```python
from build123d import *

# Parameters (mm, degrees)
F0_W     = 76.2336051654
F0_H     = 12.8238399291
F1_DEPTH = 25.4


with BuildPart() as f1:
    # F0 (on Front) → F1 (new body)
    with BuildSketch(Plane.XZ):
        with BuildLine():
            Line((0, -39.2335951328), (0, -55.1777966321))
            ThreePointArc((0, -55.1777966321), (25.3947344291, -51.0934089949), (48.2183970243, -39.2335951328))
            Line((48.2183970243, -39.2335951328), (0, -39.2335951328))
        make_face()
        Polygon((-74.7671502275, -55.1777966321), (0, -55.1777966321), (0, -39.2335951328), (-76.2336051654, -39.2335951328), (-76.2336051654, -55.1777966321), align=None)
        with BuildLine():
            Line((0, -39.2335951328), (48.2183970243, -39.2335951328))
            ThreePointArc((48.2183970243, -39.2335951328), (55.4027211148, -33.2174165852), (61.8420272475, -26.4097552037))
            Line((61.8420272475, -26.4097552037), (0, -26.4097552037))
            Line((0, -26.4097552037), (0, -39.2335951328))
        make_face()
        with BuildLine():
            ThreePointArc((-76.2336051654, -39.2335951328), (-97.2315440125, -49.2044021928), (-74.7671502275, -55.1777966321))
            Line((-74.7671502275, -55.1777966321), (-76.2336051654, -55.1777966321))
            Line((-76.2336051654, -55.1777966321), (-76.2336051654, -39.2335951328))
        make_face()
        with Locations((-38.1168025827, -32.8216751683)):
            Rectangle(F0_W, F0_H)
        with BuildLine():
            Line((61.8420272475, -13.3770994993), (61.8420272475, -26.4097552037))
            ThreePointArc((61.8420272475, -26.4097552037), (70.4948614625, -13.9048920781), (76.6509249806, 0))
            Line((76.6509249806, 0), (61.8420272475, 0))
            Line((61.8420272475, 0), (61.8420272475, -13.3770994993))
        make_face()
        Polygon((0, -26.4097552037), (61.8420272475, -26.4097552037), (61.8420272475, -13.3770994993), (0.0163518326, -13.2999842622), align=None)
        Polygon((-76.2336051654, -26.4097552037), (0, -26.4097552037), (0.0163518326, -13.2999842622), (-76.2336051654, -13.2048776019), align=None)
        Polygon((0.0163518326, -13.2999842622), (61.8420272475, -13.3770994993), (61.8420272475, 0), (21.9261534512, 0), (0.0329409185, 0), align=None)
        with BuildLine():
            ThreePointArc((-98.4511649107, 0), (-90.3999949354, -15.7771328177), (-76.2336051654, -26.4097552037))
            Line((-76.2336051654, -26.4097552037), (-76.2336051654, -13.2048776019))
            Line((-76.2336051654, -13.2048776019), (-76.2336051654, 0))
            Line((-76.2336051654, 0), (-78.4630104899, 0))
            Line((-78.4630104899, 0), (-98.4511649107, 0))
        make_face()
        Polygon((-76.2336051654, -13.2048776019), (0.0163518326, -13.2999842622), (0.0329409185, 0), (0, 0), (-20.4764902592, 0), (-61.0670559108, 0), (-76.2336051654, 0), align=None)
        Polygon((0.0329409185, 25.6056360344), (0.0329409185, 0), (21.9261534512, 0), (21.9261534512, 60.3007838378), (0.0329409185, 60.3007838378), align=None)
        Polygon((0, 0), (0.0329409185, 0), (0.0329409185, 25.6056360344), (-20.4764902592, 25.6056360344), (-20.4764902592, 0), align=None)
        Polygon((-78.4630104899, 0), (-76.2336051654, 0), (-61.0670559108, 0), (-61.0670559108, 8.4261661395), (-78.4630104899, 8.4261661395), align=None)
    extrude(amount=F1_DEPTH)


solid = f1.part
```
CAD build for the part. Positions are in the model's coordinates, mm. A direction names the side the tool comes from. Coordinates: 2 decimals unless noted, no trailing zeros. Order: outer loops, then holes, each group sorted by start corner. A loop starts at its lowest first (then second) coordinate and runs counter-clockwise, first axis right, second up. Notation, with made-up numbers: (-39.75, -33) - (-33.75, -33) arc R12 ccw to (-33.75, -18) - close; hole circle Ø5 at (-27, -3.5). An arc over 180 degrees is marked (long way). Use a Markdown table: item, result. Add a question column.
(1) Pull direction Z, two halves, no side cores. Call faces 1 (the face through (-88, -13, 0)), 2 (the face through (-12, -25.4, -26)), 3 (the face through (-97.263, -12.522, -48.783)): +Z half, -Z half, draft (parallel to the pull), parting line (faces both ways), or undercut.
(2) Saw through at B-B (y = -15). Give the cut face in (x, z), then the cut area to 3 significant figures.
(3) Saw through at D-D (z = 36.5). Give the cut face in (x, y).
(4) Saw through at C-C (x = -57). Give the cut face in (y, z), then the cut area to 3 significant figures.
(5) Flat gauge pins, fed straight in: pin 1 (1.5 mm diameter, centred on y = -20, z = -17, fed in from -X); pin 2 (2.5 mm diameter, centred on y = -14.5, z = 5.5, fed in from +X); pin 3 (5 mm diameter, centred on y = -9, z = -28, fed in from -X). Where does each tip first touch, or does it go through?
(6) Drill centre lines: line 1 along X through (y, z) = (-23.25, 3); line 2 along Z through (x, y) = (-49.5, -7.75); line 3 along Z through (x, y) = (-67, -18.75). Where is each one in solid material? Low to high. Write a range as [from, to].
(7) Which spindle directions (+Z, -Z, +X, -X, +Y, -Y) get a long thin tool onto all of the face, cutting with end or side? Do faces 4 (the face through (50, -13, 0)), 5 (the face through (-20.476, -13, 13)), 6 (the face through (-38, -13, -55.178)). Say none if no direction does.
(8) Saw through at A-A (z = 3). Give the cut face in (x, y), then the cut area to 3 significant figures.
Solved:
| question | item | result |
|---|---|---|
| 1 | face 1 | +Z half |
| 1 | face 2 | draft |
| 1 | face 3 | undercut |
| 2 | outline | (-98.45, 0) arc R39.26 ccw to (-76.23, -26.41) - (-76.23, -39.23) arc R12.38 ccw (long way) to (-74.77, -55.18) - (0, -55.18) arc R80.78 ccw to (76.65, 0) - (21.93, 0) - (21.93, 60.3) - (0.03, 60.3) - (0.03, 25.61) - (-20.48, 25.61) - (-20.48, 0) - (-61.07, 0) - (-61.07, 8.43) - (-78.46, 8.43) - (-78.46, 0) - close |
| 2 | area | 10,100 mm² |
| 3 | outline | (0.03, -25.4) - (21.93, -25.4) - (21.93, 0) - (0.03, 0) - close |
| 4 | outline | (-25.4, -55.18) - (0, -55.18) - (0, 0) - (-25.4, 0) - close |
| 4 | area | 1,400 mm² |
| 5 | pin 1 | stops at x = -90 |
| 5 | pin 2 | stops at x = 21.93 |
| 5 | pin 3 | stops at x = -78.15 |
| 6 | line 1 | x = [-78.46, -61.07], [-20.48, 21.93] |
| 6 | line 2 | z = [-55.18, 0] |
| 6 | line 3 | z = [-55.18, 8.43] |
| 7 | face 4 | +Z, +X, +Y, -Y |
| 7 | face 5 | +Z, +Y, -Y |
| 7 | face 6 | -Z, +X, +Y, -Y |
| 8 | outline | (-78.46, -25.4) - (-61.07, -25.4) - (-61.07, 0) - (-78.46, 0) - close; (-20.48, -25.4) - (21.93, -25.4) - (21.93, 0) - (-20.48, 0) - close |
| 8 | area | 1,520 mm² |
